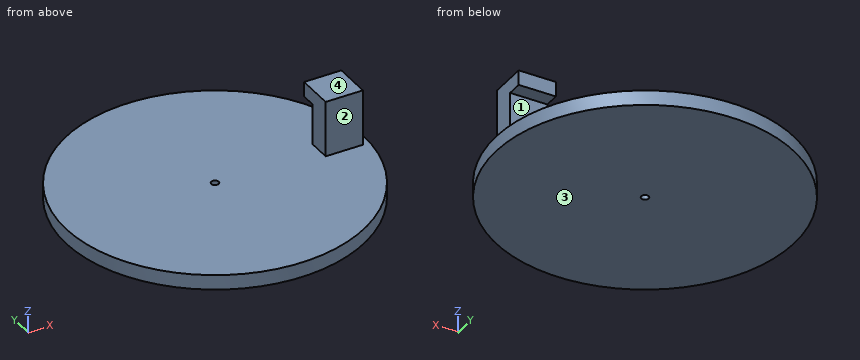
from build123d import *

# Parameters (mm, degrees)
SKETCH1_R           = 50.8
SKETCH1_R_2         = 1.27
BOSS_EXTRUDE1_DEPTH = 5.08
SKETCH2_W           = 12.7
SKETCH2_H           = 7.62
BOSS_EXTRUDE2_DEPTH = 19.05
SKETCH3_W           = 12.7
SKETCH3_H           = 5.08
BOSS_EXTRUDE3_DEPTH = 5.08


with BuildPart() as part:
    # Sketch1 → Boss-Extrude1 (new body)
    with BuildSketch(Plane.XY):
        Circle(SKETCH1_R)
        Circle(SKETCH1_R_2, mode=Mode.SUBTRACT)
    extrude(amount=BOSS_EXTRUDE1_DEPTH)

    # Sketch2 → Boss-Extrude2 (add)
    with BuildSketch(Plane.XY.offset(5.08)):
        with Locations((41.91, 0)):
            Rectangle(SKETCH2_W, SKETCH2_H)
    extrude(amount=BOSS_EXTRUDE2_DEPTH)

    # Sketch3 → Boss-Extrude3 (add)
    with BuildSketch(Plane(origin=(0, 3.81, 0), x_dir=(1, 0, 0), z_dir=(0, 1, 0))):
        with Locations((41.91, -21.59)):
            Rectangle(SKETCH3_W, SKETCH3_H)
    extrude(amount=BOSS_EXTRUDE3_DEPTH)


solid = part.part
Can you work these out from the model? Positions are in its coordinate system, mm. Face numbers are marked on the shaded views. Round coordinates to 2 decimals unless told otherwise and drop trailing zeros. Loops run counter-clockwise (first coordinate to the right, second up) from the corner with the lowest first, then second, coordinate; pieces in that order, holes last. Notation, with made-up numbers: (17, 55.25) - (30, 55.25) arc R24 cw to (30, 70.25) - close; hole circle Ø11 at (60, 49). An arc over 180 degrees is marked (long way). Answer in a Markdown table with one row per item. Add a question column.
Q1. I want a section at D-D on y = 42. List the corners of the cut face in (x, z) for me, and give its area (3 significant figures).
Q2. We'd pull the mould along Z, two halves only. Please class the marked faces 1, 2, 3 and 4: pulls with the +Z half, pulls with the -Z half, needs draft (parallel to the pull), parting line crosses it, or undercut.
Q3. I want a section at A-A on x = 0. List the corners of the cut face in (y, z) for me.
Q4. I want a section at B-B on y = 0. List the corners of the cut face in (x, z) for me, and give its area (3 significant figures).
Q5. For pin 1 Ø1.5 at (x, y) = (41.5, 7.5) entering from -Z; pin 2 Ø14 at (y, z) = (1.5, 17) entering from +X; pin 3 Ø14 at (y, z) = (2, 17) entering from -X; pin 4 Ø10 at (x, z) = (43.5, 15) entering from -Y, each with a flat end and sliding along its axis, tell me the tip position at first contact or that it passes through.
Q6. I need wall thicknesses on L1, parallel to Y at x = 0, z = 3.5; L2, parallel to Z at x = -24.5, y = -4.5; L3, parallel to X at y = -21, z = 4. Which ranges of each line are inside material? Lowest first, please.
Q7. I want a section at C-C on z = 2.75. List the corners of the cut face in (x, y) for me.
A:
| question | item | result |
|---|---|---|
| 1 | outline | (-28.58, 0) - (28.58, 0) - (28.58, 5.08) - (-28.58, 5.08) - close |
| 1 | area | 290 mm^2 |
| 2 | face 1 | undercut |
| 2 | face 2 | needs draft |
| 2 | face 3 | pulls with the -Z half |
| 2 | face 4 | pulls with the +Z half |
| 3 | outline | (-50.8, 0) - (-1.27, 0) - (-1.27, 5.08) - (-50.8, 5.08) - close; (1.27, 0) - (50.8, 0) - (50.8, 5.08) - (1.27, 5.08) - close |
| 4 | outline | (-50.8, 0) - (-1.27, 0) - (-1.27, 5.08) - (-50.8, 5.08) - close; (1.27, 0) - (50.8, 0) - (50.8, 5.08) - (48.26, 5.08) - (48.26, 24.13) - (35.56, 24.13) - (35.56, 5.08) - (1.27, 5.08) - close |
| 4 | area | 745 mm^2 |
| 5 | pin 1 | z = 0 |
| 5 | pin 2 | x = 48.26 |
| 5 | pin 3 | x = 35.56 |
| 5 | pin 4 | y = -3.81 |
| 6 | L1 | -50.8 to -1.27, 1.27 to 50.8 |
| 6 | L2 | 0 to 5.08 |
| 6 | L3 | -46.26 to 46.26 |
| 7 | outline | circle Ø101.6 at (0, 0); hole circle Ø2.54 at (0, 0) |
